```python
from build123d import *

# Parameters (mm, degrees)
SKETCH_2_R          = 52
CUT_EXTRUDE_1_DEPTH = 292
EXTRUDE_2_DEPTH     = 15
FILLET_1_R          = 10
FILLET_2_R          = 5
FILLET_3_R          = 5


with BuildPart() as part:
    # 草图1 → 旋转2 (revolve)
    with BuildSketch(Plane.XY, mode=Mode.PRIVATE) as revolve_2_sk:
        with BuildLine():
            Line((0, 0), (-124.249449603, 0))
            ThreePointArc((-124.249449603, 0), (-140.632490489, 8.528471273), (-143.043302019, 26.840402867))
            Line((-143.043302019, 26.840402867), (-60, 255))
            Line((-60, 255), (-60, 300))
            Line((-60, 300), (0, 300))
            Line((0, 300), (0, 0))
        make_face()
        with BuildLine():
            Line((-8, 8), (-124.249449603, 8))
            ThreePointArc((-124.249449603, 8), (-134.079274135, 13.117082764), (-135.525761052, 24.10424172))
            Line((-135.525761052, 24.10424172), (-52, 253.589384154))
            Line((-52, 253.589384154), (-52, 292))
            Line((-52, 292), (-8, 292))
            Line((-8, 292), (-8, 8))
        make_face(mode=Mode.SUBTRACT)
    revolve(revolve_2_sk.sketch.rotate(Axis((0, -74.77110885, 0), (0, 1, 0)), 270), axis=Axis((0, -74.77110885, 0), (0, 1, 0)))

    # 草图2 → 切除-拉伸1 (cut)
    with BuildSketch(Plane(origin=(0, 300, 0), x_dir=(1, 0, 0), z_dir=(0, 1, 0))):
        with Locations(Location((0, 0, 0), (0, 0, 90))):
            Circle(SKETCH_2_R)
    extrude(amount=-CUT_EXTRUDE_1_DEPTH, mode=Mode.SUBTRACT)

    # 草图5 → 凸台-拉伸2 (add, symmetric)
    # profile 1 of 2: a face of its own
    with BuildSketch(Plane.XY):
        with BuildLine():
            Line((-63.38666383, 234), (-96.814984609, 234))
            ThreePointArc((-96.814984609, 234), (-105.999386986, 232.17310878), (-113.785547358, 226.970562748))
            Line((-113.785547358, 226.970562748), (-168.73593113, 172.020178976))
            ThreePointArc((-168.73593113, 172.020178976), (-175.400754454, 159.217172492), (-173.51675527, 144.906777946))
            Line((-173.51675527, 144.906777946), (-129.876648813, 51.320267637))
            Line((-129.876648813, 51.320267637), (-63.38666383, 234))
        make_face()
        with BuildLine():
            ThreePointArc((-96.814984609, 230), (-104.468653256, 228.47759065), (-110.957120233, 224.142135624))
            Line((-110.957120233, 224.142135624), (-165.907504005, 169.191751851))
            ThreePointArc((-165.907504005, 169.191751851), (-171.461523442, 158.522579781), (-169.891524122, 146.597250993))
            Line((-169.891524122, 146.597250993), (-130.332580622, 61.762822889))
            Line((-130.332580622, 61.762822889), (-69.099255857, 230))
            Line((-69.099255857, 230), (-96.814984609, 230))
        make_face(mode=Mode.SUBTRACT)
    # profile 2 of 2: a face of its own
    with BuildSketch(Plane.XY):
        with BuildLine():
            Line((-69.099255857, 230), (-96.814984609, 230))
            ThreePointArc((-96.814984609, 230), (-104.468653256, 228.47759065), (-110.957120233, 224.142135624))
            Line((-110.957120233, 224.142135624), (-165.907504005, 169.191751851))
            ThreePointArc((-165.907504005, 169.191751851), (-171.461523442, 158.522579781), (-169.891524122, 146.597250993))
            Line((-169.891524122, 146.597250993), (-130.332580622, 61.762822889))
            Line((-130.332580622, 61.762822889), (-69.099255857, 230))
        make_face()
        with BuildLine():
            ThreePointArc((-96.814984609, 226), (-102.937919527, 224.78207252), (-108.128693108, 221.313708499))
            Line((-108.128693108, 221.313708499), (-163.07907688, 166.363324727))
            ThreePointArc((-163.07907688, 166.363324727), (-167.52229243, 157.82798707), (-166.266292974, 148.28772404))
            Line((-166.266292974, 148.28772404), (-130.788512431, 72.20537814))
            Line((-130.788512431, 72.20537814), (-74.811847884, 226))
            Line((-74.811847884, 226), (-96.814984609, 226))
        make_face(mode=Mode.SUBTRACT)
    extrude(amount=EXTRUDE_2_DEPTH, both=True)

    # 圆角1
    fillet_1_edges = [part.edges().sort_by_distance(p)[0] for p in [
        (-74.811847884, 226, 0),
    ]]
    fillet(fillet_1_edges, radius=FILLET_1_R)

    # 圆角2
    fillet_2_edges = [part.edges().sort_by_distance(p)[0] for p in [
        (-130.788512431, 72.20537814, 0),
    ]]
    fillet(fillet_2_edges, radius=FILLET_2_R)

    # 圆角3
    fillet_3_edges = [part.edges().sort_by_distance(p)[0] for p in [
        (-67.64337492, 234, 0),
    ]]
    fillet(fillet_3_edges, radius=FILLET_3_R)


solid = part.part
```
Input: part model. Units: mm. Frame: model coordinates. A direction names the side the tool comes from. Give positions to 0.01 mm unless a question says otherwise; leave off trailing zeros. Loops run counter-clockwise (first coordinate to the right, second up) from the corner with the lowest first, then second, coordinate; pieces in that order, holes last. Notation, with made-up numbers: M 44,27 L 88,27 A9 ccw 88,34 Z; hole C 41,4 d11. An arc over 180 degrees is marked long. Answer as CSV lines item,"result". Start each with the question number.
1. Pin query (flat end, axial travel): P1, Ø6, axis at x = -92, z = 5, coming from the -Y side; P2, Ø8, axis at x = -80.5, z = 7, coming from the +Y side; P3, Ø1, axis at x = -142, y = 101.5, coming from the -Z side; P4, Ø1, axis at x = -72.5, y = 141, coming from the +Z side. Return the tip coordinate at first contact, or that it passes through.
2. Section D-D on y = 61.5. Return loops of the section in (x, z).
3. Section A-A on y = 106. Return loops of the section in (x, z), plus the area to 3 significant figures.
4. Section B-B on x = 0. Return loops of the section in (y, z).
5. Pull-direction query (Z, two-part tool) for faces 1 (the face through (-175.364, 159.419, 0.21)), 2 (the face through (31.641, 277.12, 41.265)), 3 (the face through (89.53, 167.87, 19.88)); classes: released by +Z, released by -Z, zero draft, split by the parting line, or undercut.
6. Line query: L1, parallel to X at y = 62, z = 92; L2, parallel to X at y = 280, z = 0; L3, parallel to Z at x = -36.5, y = 213. Output: solid intervals per line, ascending.
7. Reachability of faces 4 (the face through (-100, 154, -15)), 5 (the face through (-2, 8, -2)), 6 (the face through (-100, 154, 15)) from +Z, -Z, +X, -X, +Y, -Y: full face, straight path, thin tool, end or side. Return the list, or none.
Computed values:
1,P1,"stops at y = 0"
1,P2,"stops at y = 234"
1,P3,"passes through"
1,P4,"stops at z = 71.59"
2,outline,"M -134.62,-15 L -129.56,-15 A130.43 ccw long -129.56,15 L -134.62,15 Z; hole C 0,0 d243.83"
3,outline,"M -155.37,-15 L -146.55,-15 L -146.55,15 L -155.37,15 Z; M -118.49,-15 L -113.24,-15 A114.23 ccw long -113.24,15 L -118.49,15 Z; hole C 0,0 d211.44"
3,area,"6,290 mm²"
4,outline,"M 0,-124.25 A20 ccw 26.84,-143.04 L 255,-60 L 300,-60 L 300,-52 L 253.59,-52 L 24.1,-135.53 A12 cw 8,-124.25 L 8,124.25 A12 cw 24.1,135.53 L 253.59,52 L 300,52 L 300,60 L 255,60 L 26.84,143.04 A20 ccw 0,124.25 Z"
5,face 1,"zero draft"
5,face 2,"undercut"
5,face 3,"split by the parting line"
6,L1,"x = -92.2 to -79.72, 79.72 to 92.2"
6,L2,"x = -60 to -52, 52 to 60"
6,L3,"z = -65.85 to -55.91, 55.91 to 65.85"
7,face 4,"-Z, -X, +Y"
7,face 5,"none"
7,face 6,"+Z, -X, +Y"
